The listing builds one solid part. Answer for the finished solid, in the listing's coordinates (mm). A direction names the side the tool comes from. Coordinates: 2 decimals unless noted, no trailing zeros. Loops run counter-clockwise (first coordinate to the right, second up) from the corner with the lowest first, then second, coordinate; pieces in that order, holes last. Notation, with made-up numbers: (35, -37.75) - (50, -37.75) arc R15 ccw to (50, -20.75) - close; hole circle Ø10 at (-3, -29). An arc over 180 degrees is marked (long way). Return JSON: item names as keys, results as strings. Group by question number.
1. Find the intervals of material crossed by line 1 along X through (y, z) = (0, 31.5); line 2 along X through (y, z) = (3, 9.5); line 3 along Y through (x, z) = (39.5, 41), in increasing order.
2. Which of the six approach directions +Z, -Z, +X, -X, +Y, -Y give full straight-line access (tool end or side, diameter ignored) to faces 5 (the face through (4, -53.759, 22)), 6 (the face through (0, 65.201, 40)), 7 (the face through (-0.56, 59.4, 33.39))?
3. The mould has two halves that part along Y. Classify faces 1 (the face through (-36.29, 0.24, 28)), 2 (the face through (-0.56, -59.4, 33.39)), 3 (the face through (38.964, 1.671, 27.997)), 4 (the face through (4, 53.759, 22)): pulls with the +Y half, pulls with the -Y half, needs draft (parallel to the pull), parting line crosses it, or undercut.
4. Section D-D (x = 32) is taken. Write down the section's boundary in (y, z).
5. Section A-A (z = 43) is taken. Write down the section's boundary in (x, y).
6. Section B-B (y = 0) is taken. Write down the section's boundary in (x, z).
7. Section C-C (z = 24) is taken. Write down the section's boundary in (x, y).
8. Each of these flat-tipped pins is pushed along its axis until it touches: P1, Ø12, axis at x = 8, y = -32, coming from the +Z side; P2, Ø8, axis at x = -0.5, y = -37.5, coming from the +Z side; P3, Ø8, axis at x = 8, z = 10, coming from the -Y side; P4, Ø14.5, axis at x = -30.81, y = 0, coming from the -Z side. Where does it stop, or does it pass through?
```python
from build123d import *

# Parameters (mm, degrees)
F0_W     = 87.819647
F0_H     = 93.559742
F0_R     = 4.613034
F0_R_2   = 4.621613
F1_DEPTH = 109.474
F2_R     = 28.523138
F2_R_2   = 20.412925
F3_DEPTH = 25.4
F5_W     = 138.989549
F5_H     = 60.892661
F6_DEPTH = 76.2
F7_DEPTH = 118.960742
F8_R     = 5.562192
F8_R_2   = 5.488567
F9_DEPTH = 56.790789


with BuildPart() as f1:
    # F0 (on Top) → F1 (new body)
    with BuildSketch(Plane.XY):
        with Locations((4.134112, 6.978657)):
            Rectangle(F0_W, F0_H)
        with Locations((-32.668188, 13.385462)):
            Circle(F0_R, mode=Mode.SUBTRACT)
        with Locations((36.83091, 13.385462)):
            Circle(F0_R_2, mode=Mode.SUBTRACT)
    extrude(amount=F1_DEPTH)

    # F2 (on face) → F3 (join)
    with BuildSketch(Plane.XZ.offset(39.801214)):
        with Locations((0, 61.909173)):
            Circle(F2_R)
        with Locations((0, 61.909173)):
            Circle(F2_R_2, mode=Mode.SUBTRACT)
    extrude(amount=F3_DEPTH)

    # F4: F1 across plane


with BuildPart() as f1_1:
    add(f1.part)
    add(f1.part.mirror(Plane.XZ))

    # F5 (on Front) → F6 (cut, symmetric)
    with BuildSketch(Plane.XZ):
        with Locations((8.737327, 87.23612)):
            Rectangle(F5_W, F5_H)
    extrude(amount=F6_DEPTH, both=True, mode=Mode.SUBTRACT)

    # F4_face (on face) → F7 (cut, through all)
    with BuildSketch(Plane(origin=(0, 53.758528, 50.420232), x_dir=(-1, 0, 0), z_dir=(0, 1, 0))):
        with BuildLine():
            Line((19.760552, 6.369557), (-19.760552, 6.369557))
            ThreePointArc((-19.760552, 6.369557), (0, -8.923984), (19.760552, 6.369557))
        make_face()
    extrude(amount=-F7_DEPTH, mode=Mode.SUBTRACT)

    # F8 (on Top) → F9 (cut, through all)
    with BuildSketch(Plane.XY):
        with Locations((33.658396, 0)):
            Circle(F8_R)
        with Locations((-30.80599, 0)):
            Circle(F8_R_2)
    extrude(amount=F9_DEPTH, mode=Mode.SUBTRACT)


solid = f1_1.part
```
The answers:
{
 "1": {"line 1": "x = -39.78 to -36.29, -25.32 to 28.1, 39.22 to 48.04", "line 2": "x = -39.78 to -35.4, -26.21 to 28.97, 38.34 to 48.04", "line 3": "y = -53.76 to 53.76"},
 "2": {"face 5": "-Z, -Y", "face 6": "+Z, -Z, +X, -X, +Y", "face 7": "-Z, +Y"},
 "3": {"face 1": "undercut", "face 2": "needs draft", "face 3": "undercut", "face 4": "pulls with the +Y half"},
 "4": {"outline": "(-53.76, 0) - (-5.31, 0) - (-5.31, 56.79) - (-53.76, 56.79) - close; (5.31, 0) - (53.76, 0) - (53.76, 56.79) - (5.31, 56.79) - close"},
 "5": {"outline": "(-39.78, -53.76) - (-21.35, -53.76) - (-21.35, -65.2) - (-7.69, -65.2) - (-7.69, 65.2) - (-21.35, 65.2) - (-21.35, 53.76) - (-39.78, 53.76) - close; (7.69, -65.2) - (21.35, -65.2) - (21.35, -53.76) - (48.04, -53.76) - (48.04, 53.76) - (21.35, 53.76) - (21.35, 65.2) - (7.69, 65.2) - close; hole circle Ø10.98 at (-30.81, 0); hole circle Ø11.12 at (33.66, 0)"},
 "6": {"outline": "(-39.78, 0) - (-36.29, 0) - (-36.29, 56.79) - (-39.78, 56.79) - close; (-25.32, 0) - (28.1, 0) - (28.1, 56.79) - (19.76, 56.79) arc R20.41 cw to (-19.76, 56.79) - (-25.32, 56.79) - close; (39.22, 0) - (48.04, 0) - (48.04, 56.79) - (39.22, 56.79) - close"},
 "7": {"outline": "(-39.78, -53.76) - (48.04, -53.76) - (48.04, 53.76) - (-39.78, 53.76) - close; hole circle Ø10.98 at (-30.81, 0); hole circle Ø11.12 at (33.66, 0)"},
 "8": {"P1": "stops at z = 47.05", "P2": "stops at z = 42", "P3": "stops at y = -53.76", "P4": "stops at z = 0"}
}
